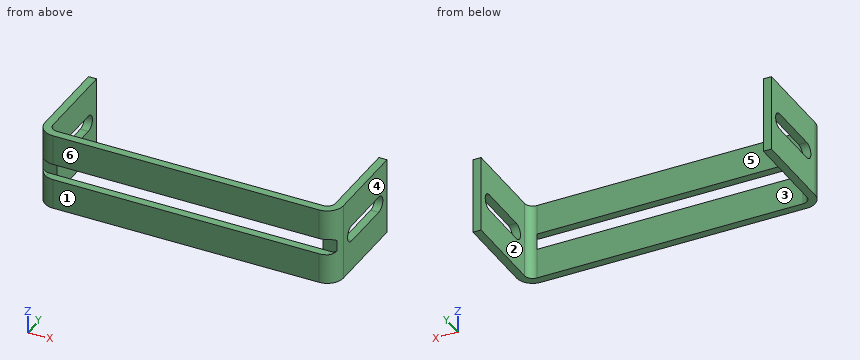
Autodesk Inventor part; units mm, degrees
ref_plane "YZ Plane" through (0, 0, 0) normal (1, 0, 0) x (0, 1, 0)
ref_plane "XZ Plane" through (0, 0, 0) normal (0, 1, 0) x (-1, 0, 0)
ref_plane "XY Plane" through (0, 0, 0) normal (0, 0, 1) x (1, 0, 0)
sketch "スケッチ1" plane through (0, 0, 0) normal (0, 1, 0) x (-1, 0, 0)
  line L0 (-37, -9.5) -> (37, -9.5)
  line L1 (37, -9.5) -> (37, 9.5)
  line L2 (37, 9.5) -> (-37, 9.5)
  line L3 (-37, 9.5) -> (-37, -9.5)
  line L4 (-37, -9.5) -> (37, 9.5) construction
  line L5 (37, -9.5) -> (-37, 9.5) construction
  point P0 (0, 0)
  dimension "d0" = 74
  dimension "d1" = 19
extrude "プレート1" add sketch "スケッチ1" along normal blind 2
sketch "スケッチ2" plane through (35, 0, -9.5) normal (1, 0, 0) x (0, 1, 0)
  line L0 (0, 19) -> (0, 0)
  line L1 (0, 0) -> (25, 0)
  line L2 (25, 0) -> (25, 19)
  line L3 (25, 19) -> (0, 19)
edge flange "フランジ1" height 25 angle 90 thickness 2 bend radius 2 thickness toward (1, 0, 0) relief tear relief width 2 relief depth 1 edges at (37, 2, 0) wall of the first edge with corners at (35, 0, 9.5) (35, 0, -9.5) (35, 25, -9.5) (35, 25, 9.5)
bend "曲げ1"
corner "コーナー1"
sketch "スケッチ3" plane through (-35, 0, 9.5) normal (-1, 0, 0) x (0, -1, 0)
  line L0 (0, -19) -> (0, 0)
  line L1 (0, 0) -> (-25, 0)
  line L2 (-25, 0) -> (-25, -19)
  line L3 (-25, -19) -> (0, -19)
edge flange "フランジ2" height 25 angle 90 thickness 2 bend radius 2 thickness toward (-1, 0, 0) relief tear relief width 2 relief depth 1 edges at (-37, 2, 0) wall of the first edge with corners at (-35, 0, -9.5) (-35, 0, 9.5) (-35, 25, 9.5) (-35, 25, -9.5)
bend "曲げ2"
corner "コーナー2"
sketch "スケッチ5" plane through (0, 0, 0) normal (0, -1, 0) x (1, 0, 0)
  arc A0 (-35, 2) -> (-35, -2) centre (-35, 0) ccw
  arc A1 (35, -2) -> (35, 2) centre (35, 0) ccw
  line L0 (-35, 2) -> (35, 2)
  line L1 (35, -2) -> (-35, -2)
  point P0 (0, 0)
  dimension "d31" = 4
  dimension "d32" = 2
  dimension "d33" = 2
  dimension "d34" = 2
  dimension "d35" = 35
  dimension "d36" = 35
extrude "押し出し1" cut sketch "スケッチ5" against normal blind 2
sketch "スケッチ6" plane through (37, 25, 9.5) normal (1, 0, 0) x (0, 0, -1)
  point P0 (9.5, -25)
sketch "スケッチ7" plane through (37, 25, 9.5) normal (1, 0, 0) x (0, 0, -1)
  line L0 (7.5, -4) -> (7.5, -17)
  arc A0 (7.5, -17) -> (11.5, -17) centre (9.5, -17) ccw
  line L1 (11.5, -17) -> (11.5, -4)
  arc A1 (11.5, -4) -> (7.5, -4) centre (9.5, -4) ccw
  line L2 (0, 0) -> (19, 0)
  line L3 (0, -21) -> (19, -21)
  point P0 (9.5, -25)
  point P1 (9.5, 0)
  dimension "d45" = 4
  dimension "d46" = 4
  dimension "d47" = 2
extrude "押し出し2" cut sketch "スケッチ7" against normal blind 100
equation "\"d2\" = Thickness"
equation "\"d3\" = BendReliefWidth"
equation "\"d4\" = BendReliefDepth"
equation "\"d5\" = MinimumRemnant"
equation "\"d6\" = TransitionRadius"
equation "\"d9\" = BendRadius"
equation "\"d10\" = CornerReliefSize"
equation "\"d11\" = GapSize"
equation "\"d12\" = JacobiRadiusSize"
equation "\"d13\" = BendReliefWidth"
equation "\"d14\" = BendReliefDepth"
equation "\"d15\" = MinimumRemnant"
equation "\"d16\" = TransitionRadius"
equation "\"d19\" = BendRadius"
equation "\"d20\" = CornerReliefSize"
equation "\"d21\" = GapSize"
equation "\"d22\" = JacobiRadiusSize"
equation "\"BendRadius\" = Thickness"
equation "\"BendReliefWidth\" = Thickness"
equation "\"BendReliefDepth\" = 0.5 * Thickness"
equation "\"CornerReliefSize\" = 4 * Thickness"
equation "\"MinimumRemnant\" = 2 * Thickness"
equation "\"TransitionRadius\" = BendRadius"
equation "\"JacobiRadiusSize\" = BendRadius"
equation "\"GapSize\" = Thickness"
properties part number "main_key_cup_col0" material "アルミニウム 6061"
Input: part model. Units: mm. Frame: model coordinates. Face numbers are marked on the shaded views. A direction names the side the tool comes from. Give positions to 0.01 mm unless a question says otherwise; leave off trailing zeros. Order: outer loops, then holes, each group sorted by start corner. A loop starts at its lowest first (then second) coordinate and runs counter-clockwise, first axis right, second up. Notation, with made-up numbers: (44.5, 59) - (95.5, 59) arc R33 ccw to (95.5, 91) - close; hole circle Ø9 at (55, 84). An arc over 180 degrees is marked (long way). Use a Markdown table: item, result.
(1) Section query B-B (y = 11.75). Output: boundary loops of the cut face in (x, z).
Computed values:
| item | result |
|---|---|
| outline | (-37, -9.5) - (-35, -9.5) - (-35, -2) - (-37, -2) - close; (-37, 2) - (-35, 2) - (-35, 9.5) - (-37, 9.5) - close; (35, -9.5) - (37, -9.5) - (37, -2) - (35, -2) - close; (35, 2) - (37, 2) - (37, 9.5) - (35, 9.5) - close |
(2) Section query A-A (z = 0). Output: boundary loops of the cut face in (x, y).
Computed values:
| item | result |
|---|---|
| outline | (-37, 4) arc R4 ccw to (-36.46, 2) - (-33, 2) arc R2 cw to (-35, 4) - (-35, 6) - (-37, 6) - close; (-37, 23) - (-35, 23) - (-35, 25) - (-37, 25) - close; (33, 2) - (36.46, 2) arc R4 ccw to (37, 4) - (37, 6) - (35, 6) - (35, 4) arc R2 cw to start; (35, 23) - (37, 23) - (37, 25) - (35, 25) - close |
(3) Line query: line 1 (X direction, y = 23, z = 3.5); line 2 (Y direction, x = -19, z = 5); line 3 (X direction, y = 3.25, z = 2). Output: solid intervals per line, ascending. Write a range as from..to.
Computed values:
| item | result |
|---|---|
| line 1 | x = -37..-35, 35..37 |
| line 2 | y = 0..2 |
| line 3 | x = -36.93..-34.85, 34.85..36.93 |
(4) Pin query (flat end, axial travel): pin 1 (6 mm diameter, centred on x = 9, z = 6, fed in from +Y); pin 2 (4 mm diameter, centred on x = 34.5, z = -0.5, fed in from -Y); pin 3 (1.7 mm diameter, centred on x = -35.5, z = 0.5, fed in from -Y). Return the tip coordinate at first contact, or that it passes through.
Computed values:
| item | result |
|---|---|
| pin 1 | stops at y = 2 |
| pin 2 | stops at y = 0 |
| pin 3 | stops at y = 2 |
(5) Section query C-C (x = 20). Output: boundary loops of the cut face in (y, z).
Computed values:
| item | result |
|---|---|
| outline | (0, -9.5) - (2, -9.5) - (2, -2) - (0, -2) - close; (0, 2) - (2, 2) - (2, 9.5) - (0, 9.5) - close |
(6) Draft query along X for the marked faces 3, 4, 5 and 6. Return one class per face: released by +X, released by -X, zero draft, split by the parting line, or undercut.
Computed values:
| item | result |
|---|---|
| face 3 | undercut |
| face 4 | released by +X |
| face 5 | undercut |
| face 6 | zero draft |
(7) Section query D-D (z = -4.5). Output: boundary loops of the cut face in (x, y).
Computed values:
| item | result |
|---|---|
| outline | (-37, 4) arc R4 ccw to (-33, 0) - (33, 0) arc R4 ccw to (37, 4) - (37, 25) - (35, 25) - (35, 4) arc R2 cw to (33, 2) - (-33, 2) arc R2 cw to (-35, 4) - (-35, 25) - (-37, 25) - close |
(8) Access query for the marked faces 1 and 2. Directions: +Z, -Z, +X, -X, +Y, -Y. A direction counts if a zero-diameter tool reaches every point of the face in a straight line with its end or side. Return the directions, or none.
Computed values:
| item | result |
|---|---|
| face 1 | +Z, -Z, +X, -X, -Y |
| face 2 | +Z, -Z, +Y |
